Work out the finished part from the listing and answer in its coordinate system (mm). Round coordinates to 2 decimals unless told otherwise and drop trailing zeros. Loops run counter-clockwise (first coordinate to the right, second up) from the corner with the lowest first, then second, coordinate; pieces in that order, holes last. Notation, with made-up numbers: (-26, -19.5) - (-5, -19.5) arc R24 cw to (-5, 8.5) - close; hole circle Ø7 at (-12.75, 61). An arc over 180 degrees is marked (long way). Answer as CSV lines item,"result". Start each with the question number.
Q1. Straight lines are drawn through the part: L1, parallel to Y at x = 3.5, z = 0; L2, parallel to Y at x = 5.5, z = -3.5; L3, parallel to Y at x = 5, z = -42. For each, find the intervals that lie inside material, in ascending order. Write a range as [from, to].
Q2. Section B-B on y = 0 is taken. Write down the section's boundary in (x, z), then the cut area to 3 significant figures.
Q3. Each of these flat-tipped pins is pushed along its axis until it touches: pin 1 Ø1.5 at (x, z) = (4, -48) entering from +Y; pin 2 Ø1 at (x, y) = (10.5, -53) entering from +Z; pin 3 Ø6 at (x, y) = (6, -15.5) entering from -Z. Where does it stop, or does it pass through?
Q4. Section D-D on y = 50 is taken. Write down the section's boundary in (x, z).
Q5. Section A-A on x = 3 is taken. Count the separate pieces of the cut face and the enclosed holes in it, then the cut area to 3 significant figures.
Q6. Section C-C on z = -27.5 is taken. Write down the section's boundary in (x, y).
Q7. The mould has two halves that part along Z. Classify faces 1 (the face through (0, -16, 1)), 2 (the face through (6, 0, -25)), 3 (the face through (5.916, -46.367, 60.47)): +Z half, -Z half, draft (parallel to the pull), parting line (faces both ways), or undercut.
```python
from build123d import *

# Parameters (mm, degrees)
SKETCH2_R           = 76.2
SKETCH2_R_2         = 2.5
SKETCH2_R_3         = 4
BOSS_EXTRUDE1_DEPTH = 12


with BuildPart() as part:
    # Sketch2 → Boss-Extrude1 (new body)
    with BuildSketch(Plane(origin=(0, 0, 0), x_dir=(0, 0, -1), z_dir=(1, 0, 0))):
        Circle(SKETCH2_R)
        with Locations((0, 27.5)):
            Circle(SKETCH2_R_2, mode=Mode.SUBTRACT)
        with Locations((27.5, 0)):
            Circle(SKETCH2_R_2, mode=Mode.SUBTRACT)
        with Locations((0, -27.5)):
            Circle(SKETCH2_R_2, mode=Mode.SUBTRACT)
        with Locations((-27.5, 0)):
            Circle(SKETCH2_R_2, mode=Mode.SUBTRACT)
        with Locations((0, 50)):
            Circle(SKETCH2_R_3, mode=Mode.SUBTRACT)
        with Locations((43.301270189, -25)):
            Circle(SKETCH2_R_3, mode=Mode.SUBTRACT)
        with Locations((-43.301270189, -25)):
            Circle(SKETCH2_R_3, mode=Mode.SUBTRACT)
        Circle(SKETCH2_R_3, mode=Mode.SUBTRACT)
    extrude(amount=BOSS_EXTRUDE1_DEPTH)


solid = part.part
```
Findings:
1,L1,"y = [-76.2, -30], [-25, -4], [4, 25], [30, 46], [54, 76.2]"
1,L2,"y = [-76.12, -1.94], [1.94, 48.06], [51.94, 76.12]"
1,L3,"y = [-63.58, -28.78], [-21.22, 63.58]"
2,outline,"(0, -76.2) - (12, -76.2) - (12, -30) - (0, -30) - close; (0, -25) - (12, -25) - (12, -4) - (0, -4) - close; (0, 4) - (12, 4) - (12, 25) - (0, 25) - close; (0, 30) - (12, 30) - (12, 76.2) - (0, 76.2) - close"
2,area,"1,610 mm^2"
3,pin 1,"stops at y = 59.78"
3,pin 2,"stops at z = 55.23"
3,pin 3,"stops at z = -75.17"
4,outline,"(0, -57.5) - (12, -57.5) - (12, -4) - (0, -4) - close; (0, 4) - (12, 4) - (12, 57.5) - (0, 57.5) - close"
5,separate pieces,"1"
5,enclosed holes,"8"
5,area,"18,000 mm^2"
6,outline,"(0, -71.06) - (12, -71.06) - (12, -2.5) - (0, -2.5) - close; (0, 2.5) - (12, 2.5) - (12, 71.06) - (0, 71.06) - close"
7,face 1,"draft"
7,face 2,"undercut"
7,face 3,"parting line"
